Can you work these out from the model? Positions are in its coordinate system, mm. Face numbers are marked on the shaded views. A direction names the side the tool comes from. Give positions to 0.01 mm unless a question says otherwise; leave off trailing zeros. Write each loop counter-clockwise with the first axis right and the second up, starting at its lowest first coordinate (ties: lowest second). Pieces come first, ordered by that corner, then holes. Notation, with made-up numbers: (-5.75, 57.5) -> (53.25, 57.5) arc R24 cw to (53.25, 70.5) -> close; hole circle Ø10 at (81, -16.75). An arc over 180 degrees is marked (long way). Answer as CSV lines item,"result". Start each with the question number.
1. If we section it at A-A on x = 19.05: Write out the boundary of the cut face in (y, z) (3 decimals).
2. I need wall thicknesses on line 1 (Z direction, x = 35.7, y = -38.1) (3 decimals); line 2 (Z direction, x = 33.5, y = -25); line 3 (X direction, y = -52, z = 54). Which ranges of each line are inside material? Lowest first, please. Write a range as [from, to].
3. If we section it at C-C on z = 38.1: Count the separate pieces of the cut face and the enclosed holes in it, plus the area to 3 significant figures.
4. I'm going to push flat-ended pins straight in: P1, Ø7.5, axis at y = -88.9, z = 57.15, coming from the -X side; P2, Ø7.5, axis at x = 19.05, y = -38.1, coming from the +Z side. Where does each tip first touch, or does it pass through?
5. If we section it at B-B on y = -107: Write out the boundary of the cut face in (x, z), plus the area to 3 significant figures.
6. If we section it at D-D on x = -28: Write out the boundary of the cut face in (y, z).
7. On a 3-axis mill with a long thin cutter (end or side, diameter ignored), from which of +Z, -Z, +X, -X, +Y, -Y can I reach the whole of each face in a straight line? I mean the marked faces 1 and 2. Say none if no direction works.
8. If we mould it in two halves opening along Z, with no side actions, what happens to the marked faces 3, 4 and 5? For each: pulls with the +Z half, pulls with the -Z half, needs draft (parallel to the pull), parting line crosses it, or undercut.
```python
from build123d import *

# Parameters (mm, degrees)
F3_DEPTH       = 152.4
F1_R           = 6.35
F4_DEPTH       = 152.4
F2_R           = 2.032
F5_DEPTH       = 152.401
F6_R           = 3.175
F7_DEPTH       = 38.101
F7_DEPTH_BACK  = 38.101
F8_R           = 3.175
F9_DEPTH       = 76.201
F11_DEPTH      = 38.101
F11_DEPTH_BACK = 38.101
F13_DEPTH      = 76.201


with BuildPart() as f3:
    # F0 (on Front) → F3 (new body)
    with BuildSketch(Plane.XZ):
        Polygon((-38.1, 76.2), (-38.1, 0), (38.1, 0), (38.1, 76.2), (33.02, 76.2), (33.02, 5.08), (-33.02, 5.08), (-33.02, 76.2), align=None)
    extrude(amount=F3_DEPTH)

    # F1 (on Front) → F4 (join)
    with BuildSketch(Plane.XZ):
        with Locations((-31.75, 6.35)):
            Circle(F1_R)
        with Locations((31.75, 6.35)):
            Circle(F1_R)
        with Locations((-31.75, 69.85)):
            Circle(F1_R)
        with Locations((31.75, 69.85)):
            Circle(F1_R)
    extrude(amount=F4_DEPTH)

    # F2 (on Front) → F5 (cut, through all)
    with BuildSketch(Plane.XZ):
        with Locations((-31.75, 69.85)):
            Circle(F2_R)
        with Locations((31.75, 69.85)):
            Circle(F2_R)
        with Locations((-31.75, 6.35)):
            Circle(F2_R)
        with Locations((31.75, 6.35)):
            Circle(F2_R)
    extrude(amount=F5_DEPTH, mode=Mode.SUBTRACT)

    # F6 (on Right) → F7 (cut, two sides)
    with BuildSketch(Plane.YZ) as f7_sk:
        with Locations((-12.7, 19.05)):
            Circle(F6_R)
        with Locations((-12.7, 38.1)):
            Circle(F6_R)
        with Locations((-12.7, 57.15)):
            Circle(F6_R)
        with Locations((-38.1, 19.05)):
            Circle(F6_R)
        with Locations((-38.1, 38.1)):
            Circle(F6_R)
        with Locations((-38.1, 57.15)):
            Circle(F6_R)
        with Locations((-63.5, 19.05)):
            Circle(F6_R)
        with Locations((-63.5, 38.1)):
            Circle(F6_R)
        with Locations((-63.5, 57.15)):
            Circle(F6_R)
        with Locations((-88.9, 19.05)):
            Circle(F6_R)
        with Locations((-88.9, 38.1)):
            Circle(F6_R)
        with Locations((-88.9, 57.15)):
            Circle(F6_R)
        with Locations((-114.3, 19.05)):
            Circle(F6_R)
        with Locations((-114.3, 38.1)):
            Circle(F6_R)
        with Locations((-114.3, 57.15)):
            Circle(F6_R)
        with Locations((-139.7, 19.05)):
            Circle(F6_R)
        with Locations((-139.7, 38.1)):
            Circle(F6_R)
        with Locations((-139.7, 57.15)):
            Circle(F6_R)
    extrude(amount=-F7_DEPTH, mode=Mode.SUBTRACT)
    extrude(f7_sk.sketch, amount=F7_DEPTH_BACK, mode=Mode.SUBTRACT)

    # F8 (on Top) → F9 (cut, through all)
    with BuildSketch(Plane.XY):
        with Locations((-19.05, -12.7)):
            Circle(F8_R)
        with Locations((-19.05, -38.1)):
            Circle(F8_R)
        with Locations((-19.05, -63.5)):
            Circle(F8_R)
        with Locations((-19.05, -88.9)):
            Circle(F8_R)
        with Locations((0, -12.7)):
            Circle(F8_R)
        with Locations((0, -38.1)):
            Circle(F8_R)
        with Locations((0, -63.5)):
            Circle(F8_R)
        with Locations((0, -88.9)):
            Circle(F8_R)
        with Locations((19.05, -12.7)):
            Circle(F8_R)
        with Locations((19.05, -38.1)):
            Circle(F8_R)
        with Locations((19.05, -63.5)):
            Circle(F8_R)
        with Locations((19.05, -88.9)):
            Circle(F8_R)
        with Locations((-19.05, -114.3)):
            Circle(F8_R)
        with Locations((-19.05, -139.7)):
            Circle(F8_R)
        with Locations((0, -114.3)):
            Circle(F8_R)
        with Locations((0, -139.7)):
            Circle(F8_R)
        with Locations((19.05, -114.3)):
            Circle(F8_R)
        with Locations((19.05, -139.7)):
            Circle(F8_R)
    extrude(amount=F9_DEPTH, mode=Mode.SUBTRACT)

    # F10 (on Right) → F11 (cut, two sides)
    with BuildSketch(Plane.YZ) as f11_sk:
        with BuildLine():
            Line((0, 44.45), (0, 50.8))
            Line((0, 50.8), (-3.175, 50.8))
            ThreePointArc((-3.175, 50.8), (-6.35, 47.625), (-3.175, 44.45))
            Line((-3.175, 44.45), (0, 44.45))
        make_face()
        with BuildLine():
            Line((0, 25.4), (0, 31.75))
            Line((0, 31.75), (-3.175, 31.75))
            ThreePointArc((-3.175, 31.75), (-6.35, 28.575), (-3.175, 25.4))
            Line((-3.175, 25.4), (0, 25.4))
        make_face()
    extrude(amount=-F11_DEPTH, mode=Mode.SUBTRACT)
    extrude(f11_sk.sketch, amount=F11_DEPTH_BACK, mode=Mode.SUBTRACT)

    # F12 (on Top) → F13 (cut, through all)
    with BuildSketch(Plane.XY):
        with BuildLine():
            Line((-6.35, 0), (-12.7, 0))
            Line((-12.7, 0), (-12.7, -3.175))
            ThreePointArc((-12.7, -3.175), (-9.525, -6.35), (-6.35, -3.175))
            Line((-6.35, -3.175), (-6.35, 0))
        make_face()
        with BuildLine():
            Line((12.7, 0), (6.35, 0))
            Line((6.35, 0), (6.35, -3.175))
            ThreePointArc((6.35, -3.175), (9.525, -6.35), (12.7, -3.175))
            Line((12.7, -3.175), (12.7, 0))
        make_face()
    extrude(amount=F13_DEPTH, mode=Mode.SUBTRACT)


solid = f3.part
```
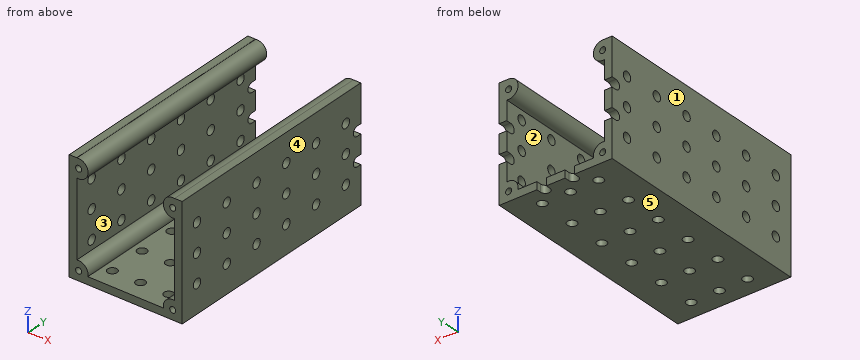
Computed values:
1,outline,"(-152.4, 0) -> (-142.875, 0) -> (-142.875, 5.08) -> (-152.4, 5.08) -> close; (-136.525, 0) -> (-117.475, 0) -> (-117.475, 5.08) -> (-136.525, 5.08) -> close; (-111.125, 0) -> (-92.075, 0) -> (-92.075, 5.08) -> (-111.125, 5.08) -> close; (-85.725, 0) -> (-66.675, 0) -> (-66.675, 5.08) -> (-85.725, 5.08) -> close; (-60.325, 0) -> (-41.275, 0) -> (-41.275, 5.08) -> (-60.325, 5.08) -> close; (-34.925, 0) -> (-15.875, 0) -> (-15.875, 5.08) -> (-34.925, 5.08) -> close; (-9.525, 0) -> (0, 0) -> (0, 5.08) -> (-9.525, 5.08) -> close"
2,line 1,"z = [0, 15.875], [22.225, 34.925], [41.275, 53.975], [60.325, 76.2]"
2,line 2,"z = [0, 5.32], [7.38, 68.82], [70.88, 76.2]"
2,line 3,"x = [-38.1, -33.02], [33.02, 38.1]"
3,separate pieces,"14"
3,enclosed holes,"0"
3,area,"1,160 mm2"
4,P1,"stops at x = -38.1"
4,P2,"stops at z = 5.08"
5,outline,"(-38.1, 0) -> (38.1, 0) -> (38.1, 76.2) -> (33.02, 76.2) -> (33.02, 76.07) arc R6.35 ccw (long way) to (33.02, 63.63) -> (33.02, 12.57) arc R6.35 ccw to (25.53, 5.08) -> (-25.53, 5.08) arc R6.35 ccw to (-33.02, 12.57) -> (-33.02, 63.63) arc R6.35 ccw (long way) to (-33.02, 76.07) -> (-33.02, 76.2) -> (-38.1, 76.2) -> close; hole circle Ø4.06 at (-31.75, 6.35); hole circle Ø4.06 at (-31.75, 69.85); hole circle Ø4.06 at (31.75, 6.35); hole circle Ø4.06 at (31.75, 69.85)"
5,area,"1,320 mm2"
6,outline,"(-152.4, 0) -> (0, 0) -> (0, 11.47) -> (-152.4, 11.47) -> close; (-152.4, 64.73) -> (0, 64.73) -> (0, 74.97) -> (-152.4, 74.97) -> close"
7,face 1,"+Z, -Z, -X, +Y, -Y"
7,face 2,"+Y, -Y"
8,face 3,"undercut"
8,face 4,"needs draft"
8,face 5,"pulls with the -Z half"
